The listing builds one solid part. Answer for the finished solid, in the listing's coordinates (mm). Face numbers are marked on the shaded views. A direction names the side the tool comes from. Give positions to 0.01 mm unless a question says otherwise; leave off trailing zeros. Loops run counter-clockwise (first coordinate to the right, second up) from the corner with the lowest first, then second, coordinate; pieces in that order, holes last. Notation, with made-up numbers: M 45.5,85.5 L 79.5,85.5 A10 ccw 79.5,92.5 Z; hole C 8.5,48.25 d11. An arc over 180 degrees is marked long. Return JSON: item names as keys, results as strings.
from build123d import *

# Parameters (mm, degrees)
SALIENTE_EXTRUIR1_DEPTH = 15
CROQUIS2_R              = 2.5
SALIENTE_EXTRUIR2_DEPTH = 1
CROQUIS3_W              = 12
CROQUIS3_H              = 9.99
SALIENTE_EXTRUIR3_DEPTH = 9
REDONDEO1_R             = 0.2
CROQUIS4_R              = 1.95
SALIENTE_EXTRUIR4_DEPTH = 0.6
SALIENTE_EXTRUIR5_DEPTH = 9.27
CHAFL_N1_SIZE           = 0.2
CROQUIS6_R              = 0.5
CORTAR_EXTRUIR1_DEPTH   = 2


with BuildPart() as part:
    # Croquis1 → Saliente-Extruir1 (new body)
    with BuildSketch(Plane.XY):
        with BuildLine():
            Line((-3.5, -5), (3.5, -5))
            ThreePointArc((3.5, -5), (6.019255673, 0), (3.5, 5))
            Line((3.5, 5), (-3.5, 5))
            ThreePointArc((-3.5, 5), (-5.980744327, 0), (-3.5, -5))
        make_face()
    extrude(amount=SALIENTE_EXTRUIR1_DEPTH)

    # Croquis2 → Saliente-Extruir2 (add)
    with BuildSketch(Plane(origin=(0, 0, 0), x_dir=(-1, 0, 0), z_dir=(0, 0, -1))):
        Circle(CROQUIS2_R)
    extrude(amount=SALIENTE_EXTRUIR2_DEPTH)

    # Croquis3 → Saliente-Extruir3 (add)
    with BuildSketch(Plane.XY.offset(15)):
        Rectangle(CROQUIS3_W, CROQUIS3_H)
    extrude(amount=SALIENTE_EXTRUIR3_DEPTH)

    # Redondeo1
    redondeo1_edges = [part.edges().sort_by_distance(p)[0] for p in [
        (6, -4.995, 19.5),
        (6, 4.995, 19.5),
        (-6, 4.995, 19.5),
        (-6, -4.995, 19.5),
    ]]
    fillet(redondeo1_edges, radius=REDONDEO1_R)

    # Croquis4 → Saliente-Extruir4 (add)
    with BuildSketch(Plane.XY.offset(24)):
        Circle(CROQUIS4_R)
    extrude(amount=SALIENTE_EXTRUIR4_DEPTH)

    # Croquis5 → Saliente-Extruir5 (add)
    with BuildSketch(Plane.XY.offset(24.6)):
        with BuildLine():
            Line((-1.118033989, 1), (1.118033989, 1))
            ThreePointArc((1.118033989, 1), (0, -1.5), (-1.118033989, 1))
        make_face()
    extrude(amount=SALIENTE_EXTRUIR5_DEPTH)

    # Chaflán1
    chafl_n1_edges = [part.edges().sort_by_distance(p)[0] for p in [
        (0, -1.5, 33.87),
    ]]
    chamfer(chafl_n1_edges, length=CHAFL_N1_SIZE)

    # Croquis6 → Cortar-Extruir1 (cut)
    with BuildSketch(Plane.XY.offset(24)):
        with Locations((-4.5, 0)):
            Circle(CROQUIS6_R)
        with Locations((4.5, 0)):
            Circle(CROQUIS6_R)
    extrude(amount=-CORTAR_EXTRUIR1_DEPTH, mode=Mode.SUBTRACT)


solid = part.part
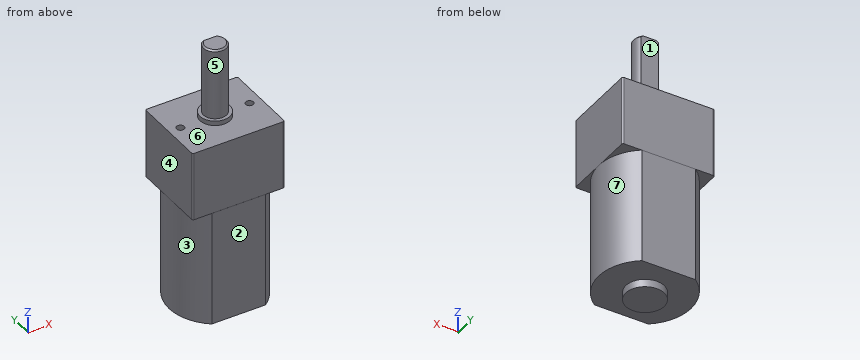
(1) Straight lines are drawn through the part: line 1 along Y through (x, z) = (4.5, 23) (3 decimals); line 2 along X through (y, z) = (-1.5, 23.5); line 3 along Z through (x, y) = (-4.75, -0.25). For each, find the intervals that lie inside material, in ascending order.
Values follow:
{"line 1": "-4.995 to -0.5, 0.5 to 4.995", "line 2": "-6 to 6", "line 3": "0 to 22"}
(2) The part is cut by section C-C (x = 0). Determine the outline of the cut face in (y, z) (3 decimals), and give its area (3 significant figures).
Values follow:
{"outline": "M -5,0 L -2.5,0 L -2.5,-1 L 2.5,-1 L 2.5,0 L 5,0 L 5,15 L 4.995,15 L 4.995,24 L 1.95,24 L 1.95,24.6 L 1,24.6 L 1,33.87 L -1.3,33.87 L -1.5,33.67 L -1.5,24.6 L -1.95,24.6 L -1.95,24 L -4.995,24 L -4.995,15 L -5,15 Z", "area": "270 mm²"}
(3) Determine the mould class of the marked faces 4, 5, 6 and 7 for opening direction X: released by +X, released by -X, zero draft, split by the parting line, or undercut.
Values follow:
{"face 4": "released by -X", "face 5": "split by the parting line", "face 6": "zero draft", "face 7": "released by +X"}
(4) The part is cut by section D-D (z = 29). Determine the outline of the cut face in (x, y).
Values follow:
{"outline": "M -1.12,1 A1.5 ccw long 1.12,1 Z"}
(5) Given pin 1 (1.2 mm diameter, centred on x = -5, y = -2.5, fed in from -Z); pin 2 (6 mm diameter, centred on y = 0.5, z = 21, fed in from +X); pin 3 (1.5 mm diameter, centred on y = 0, z = 14, fed in from -X), each flat-ended and moving along its own axis, determine where each tip first touches the part or whether it passes through.
Values follow:
{"pin 1": "z = 0", "pin 2": "x = 6", "pin 3": "x = -5.98"}
(6) A tool of negligible diameter and unlimited length cuts with its end or side. For the marked faces 1, 2 and 3, from which of +Z, -Z, +X, -X, +Y, -Y can it reach the whole face along a straight path? Write none if from no direction.
Values follow:
{"face 1": "+Z, +X, -X, +Y", "face 2": "+Z, -Z, +X, -X, -Y", "face 3": "-Z, -X"}
(7) The part is cut by section A-A (z = 23). Determine the outline of the cut face in (x, y) (3 decimals).
Values follow:
{"outline": "M -6,-4.795 A0.2 ccw -5.8,-4.995 L 5.8,-4.995 A0.2 ccw 6,-4.795 L 6,4.795 A0.2 ccw 5.8,4.995 L -5.8,4.995 A0.2 ccw -6,4.795 Z; hole C -4.5,0 d1; hole C 4.5,0 d1"}
